```python
from build123d import *

# Parameters (mm, degrees)
SKETCH1_W                      = 215.9
SKETCH1_H                      = 130
BOSS_EXTRUDE1_DEPTH            = 6
FILLET1_R                      = 5.5118
CAVITY3_DEPTH                  = 3
CBORE_FOR_M4_SHCS1_D           = 4.8
CBORE_FOR_M4_SHCS1_CBORE_D     = 8
CBORE_FOR_M4_SHCS1_CBORE_DEPTH = 4


# Read off the part's stored shape, not the designer's step: Cavity3
with BuildPart() as part:
    # Sketch1 → Boss-Extrude1 (new body)
    with BuildSketch(Plane(origin=(0, 0, 0), x_dir=(1, 0, 0), z_dir=(0, 1, 0))):
        Rectangle(SKETCH1_W, SKETCH1_H)
    extrude(amount=BOSS_EXTRUDE1_DEPTH)

    # Fillet1
    fillet1_edges = [part.edges().sort_by_distance(p)[0] for p in [
        (107.95, 3, 65),
        (-107.95, 3, 65),
        (-107.95, 3, -65),
        (107.95, 3, -65),
    ]]
    fillet(fillet1_edges, radius=FILLET1_R)

    # Cavity3 outline → Cavity3 (cut)
    with BuildSketch(Plane(origin=(0, 0, 0), x_dir=(1, 0, 0), z_dir=(0, 1, 0))):
        with BuildLine():
            ThreePointArc((-106.1, -52.4764), (-105.807106781, -53.183506781), (-105.1, -53.4764))
            Line((-105.1, -53.4764), (-101.9382, -53.4764))
            ThreePointArc((-101.9382, -53.4764), (-98.040768843, -55.090768843), (-96.4264, -58.9882))
            Line((-96.4264, -58.9882), (-96.4264, -62.65))
            ThreePointArc((-96.4264, -62.65), (-96.133506781, -63.357106781), (-95.4264, -63.65))
            Line((-95.4264, -63.65), (95.4264, -63.65))
            ThreePointArc((95.4264, -63.65), (96.133506781, -63.357106781), (96.4264, -62.65))
            Line((96.4264, -62.65), (96.4264, -58.9882))
            ThreePointArc((96.4264, -58.9882), (98.040768843, -55.090768843), (101.9382, -53.4764))
            Line((101.9382, -53.4764), (105.1, -53.4764))
            ThreePointArc((105.1, -53.4764), (105.807106781, -53.183506781), (106.1, -52.4764))
            Line((106.1, -52.4764), (106.1, 52.4764))
            ThreePointArc((106.1, 52.4764), (105.807106781, 53.183506781), (105.1, 53.4764))
            Line((105.1, 53.4764), (104.8, 53.4764))
            Line((104.8, 53.4764), (104.8, -52.4764))
            Line((104.8, -52.4764), (101.4264, -52.4764))
            ThreePointArc((101.4264, -52.4764), (97.183759313, -54.233759313), (95.4264, -58.4764))
            Line((95.4264, -58.4764), (95.4264, -62.35))
            Line((95.4264, -62.35), (-95.4264, -62.35))
            Line((-95.4264, -62.35), (-95.4264, -58.4764))
            ThreePointArc((-95.4264, -58.4764), (-97.183759313, -54.233759313), (-101.4264, -52.4764))
            Line((-101.4264, -52.4764), (-104.8, -52.4764))
            Line((-104.8, -52.4764), (-104.8, 52.4764))
            Line((-104.8, 52.4764), (-101.4264, 52.4764))
            ThreePointArc((-101.4264, 52.4764), (-97.183759313, 54.233759313), (-95.4264, 58.4764))
            Line((-95.4264, 58.4764), (-95.4264, 62.35))
            Line((-95.4264, 62.35), (96.4264, 62.35))
            Line((96.4264, 62.35), (96.4264, 62.65))
            ThreePointArc((96.4264, 62.65), (96.133506781, 63.357106781), (95.4264, 63.65))
            Line((95.4264, 63.65), (-95.4264, 63.65))
            ThreePointArc((-95.4264, 63.65), (-96.133506781, 63.357106781), (-96.4264, 62.65))
            Line((-96.4264, 62.65), (-96.4264, 58.9882))
            ThreePointArc((-96.4264, 58.9882), (-98.040768843, 55.090768843), (-101.9382, 53.4764))
            Line((-101.9382, 53.4764), (-105.1, 53.4764))
            ThreePointArc((-105.1, 53.4764), (-105.807106781, 53.183506781), (-106.1, 52.4764))
            Line((-106.1, 52.4764), (-106.1, -52.4764))
        make_face()
        with BuildLine():
            Line((95.4264, 52.4764), (101.4264, 52.4764))
            ThreePointArc((101.4264, 52.4764), (97.183759313, 54.233759313), (95.4264, 58.4764))
            Line((95.4264, 58.4764), (95.4264, 52.4764))
        make_face()
    extrude(amount=CAVITY3_DEPTH, mode=Mode.SUBTRACT)

    # CBORE for M4 SHCS1 (through all)
    with Locations(Plane(origin=(0, 6, 0), x_dir=(1, 0, 0), z_dir=(0, 1, 0))):
        with Locations((-101.9382, 58.9882), (-101.9382, -58.9882), (101.9382, -58.9882), (101.9382, 58.9882)):
            CounterBoreHole(CBORE_FOR_M4_SHCS1_D / 2, CBORE_FOR_M4_SHCS1_CBORE_D / 2, CBORE_FOR_M4_SHCS1_CBORE_DEPTH)


solid = part.part
```
Geometry check sheet. Reference: the model listing, model coordinates, mm. A direction names the side the tool comes from. Coordinates: 2 decimals unless noted, no trailing zeros.
Item 1: Sectioned sample at A-A, the plane y = 1.1. Count the separate pieces of the cut face and the enclosed holes in it, then the cut area to 3 significant figures.
Item 2: Access from +Z, -Z, +X, -X, +Y, -Y to the whole of each face (thin tool, end or side, straight path). Record for faces 4 (the face through (-100, 2, 61)), 5 (the face through (98, 1.48, 55.13)), 6 (the face through (106.38, 3.04, -63.34)).
Item 3: Go/stop test with flat-tipped pins: pin 1 Ø3.5 at (y, z) = (1, -61.5) entering from +X; pin 2 Ø0.9 at (y, z) = (1.5, 60.5) entering from -X; pin 3 Ø6.5 at (x, z) = (102, -59) entering from +Y. Record where each tip stops, or that it passes through.
Item 4: Release check for a two-part mould opening along X. For faces 1 (the face through (-1, 3, 65)), 2 (the face through (106.29, 3.04, 63.43)), 3 (the face through (-97.14, 1.48, 54.28)) record: released by +X, released by -X, zero draft, split by the parting line, or undercut.
Item 5: Thickness scan on line 1 (X direction, y = 0.3, z = -2); line 2 (Z direction, x = -95, y = 0.65). Record the ranges inside material, lowest first.
Check result:
1. separate pieces: 1
1. enclosed holes: 6
1. area: 27,100 mm2
2. face 4: +Y
2. face 5: -Y
2. face 6: -Z, +X, +Y, -Y
3. pin 1: stops at x = 107.94
3. pin 2: stops at x = -107.92
3. pin 3: stops at y = 2
4. face 1: zero draft
4. face 2: released by +X
4. face 3: undercut
5. line 1: x = -107.95 to -106.1, -104.8 to 104.8, 106.1 to 107.95
5. line 2: z = -65 to -63.65, -62.35 to 62.35, 63.65 to 65
